For this review, use the dimensioned drawing (mm, ordinates from the lowest corner) and the shaded views. Coordinates: 2 decimals unless noted, no trailing zeros. Write each loop counter-clockwise with the first axis right and the second up, starting at its lowest first coordinate (ties: lowest second). Pieces come first, ordered by that corner, then holes.
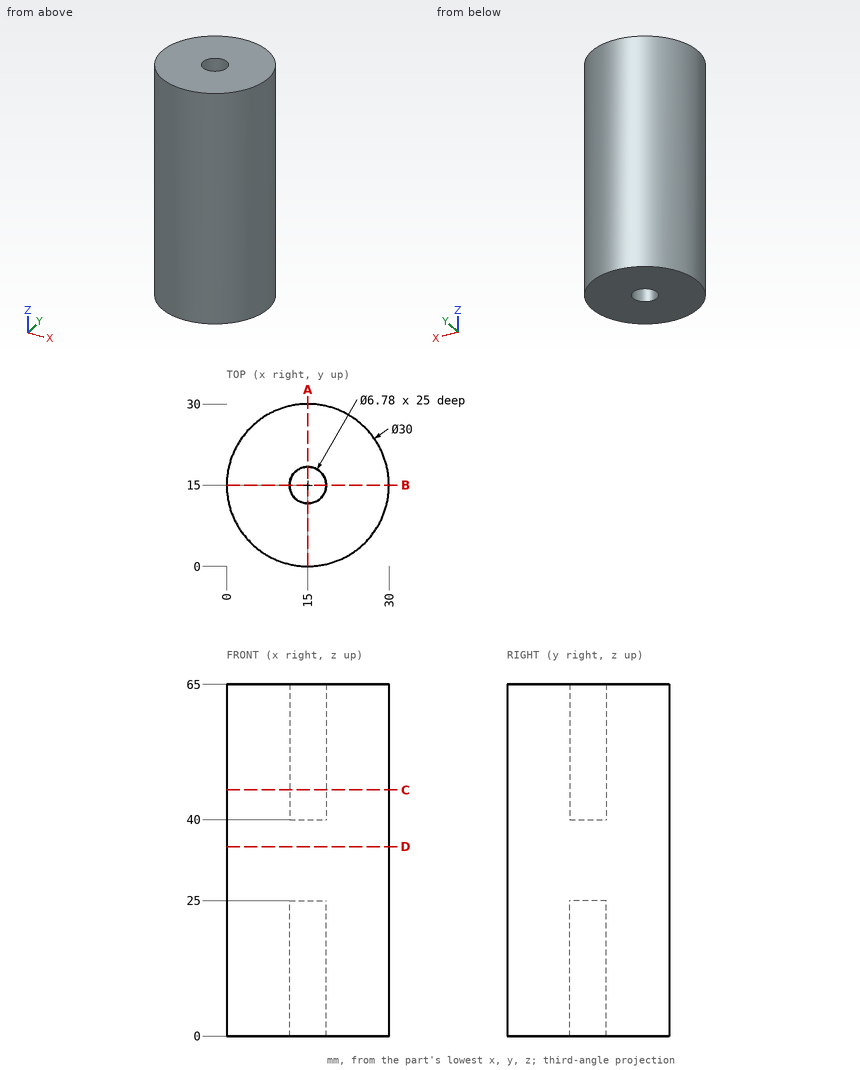
(1) Consider section C-C (z = 45.5). Give the boundary of the cut face in (x, y), plus the area to 3 significant figures.
(2) Consider section D-D (z = 35). Give the boundary of the cut face in (x, y), plus the area to 3 significant figures.
(3) Insertion check: pin 1 Ø12 at (x, z) = (3.5, 22) entering from -Y; pin 2 Ø8 at (x, z) = (8.5, 57.5) entering from +Y; pin 3 Ø5.5 at (x, y) = (15, 15) entering from -Z. Each pin has a flat end and moves straight along its axis. Give the tip position at first contact, or say it passes through.
(4) Wall thickness on line 1 (Y direction, x = 15, z = 49.5); line 2 (Z direction, x = 18, y = 13.5); line 3 (X direction, y = 11.75, z = 36.5): over which ranges is each line inside the solid? List them lowest first.
(5) Consider section A-A (x = 15). Give the boundary of the cut face in (y, z), plus the area to 3 significant figures.
Results:
1. outline: circle Ø30 at (15, 15); hole circle Ø6.78 at (15, 15)
1. area: 671 mm2
2. outline: circle Ø30 at (15, 15)
2. area: 707 mm2
3. pin 1: stops at y = 1.04
3. pin 2: stops at y = 29.79
3. pin 3: stops at z = 25
4. line 1: y = 0 to 11.61, 18.39 to 30
4. line 2: z = 25 to 40
4. line 3: x = 0.36 to 29.64
5. outline: (0, 0) - (11.61, 0) - (11.61, 25) - (18.39, 25) - (18.39, 0) - (30, 0) - (30, 65) - (18.39, 65) - (18.39, 40) - (11.61, 40) - (11.61, 65) - (0, 65) - close
5. area: 1,610 mm2
